For this review, take the finished solid that the model builds, in its own axes (mm). Face numbers are marked on the shaded views. A direction names the side the tool comes from. Give positions to 0.01 mm unless a question says otherwise; leave off trailing zeros. Write each loop counter-clockwise with the first axis right and the second up, starting at its lowest first coordinate (ties: lowest second). Pieces come first, ordered by that corner, then holes.
Q1. We need section B-B (z = 0). Write out the cut boundary in (x, y), then the cut area to 3 significant figures.
Q2. We need section A-A (x = 0). Write out the cut boundary in (y, z).
Q3. We need section C-C (y = -8.75). Write out the cut boundary in (x, z).
Q4. Machinability: for the marked faces 4, 5 and 6, which of the approach directions +Z, -Z, +X, -X, +Y, -Y give a long, thin tool a straight path to every point of the face, cutting with its end or side? Answer none if there is none.
Q5. For line 1 (Y direction, x = -1.3, z = -0.05); line 2 (Z direction, x = -0.1, y = -8); line 3 (Y direction, x = 1.35, z = 0.9), list the stretches that pass through material, from the lowest coordinate up.
Q6. Insertion check: P1, Ø2, axis at y = -8, z = -2, coming from the -X side; P2, Ø1.1, axis at y = 1.5, z = -1, coming from the -X side; P3, Ø1.1, axis at x = 1, y = 1.5, coming from the -Z side. Each pin has a flat end and moves straight along its axis. Give the tip position at first contact, or say it passes through.
Q7. Mouldability with a two-part tool opening along Z and no side actions: class the marked faces 1, 2 and 3 as released by +Z, released by -Z, zero draft, split by the parting line, or undercut.
Autodesk Inventor part; units mm, degrees
ref_plane "YZ Plane" through (0, 0, 0) normal (1, 0, 0) x (0, 1, 0)
ref_plane "XZ Plane" through (0, 0, 0) normal (0, 1, 0) x (-1, 0, 0)
ref_plane "XY Plane" through (0, 0, 0) normal (0, 0, 1) x (1, 0, 0)
sketch "Skizze1" plane through (0, 0, 0) normal (0, 1, 0) x (-1, 0, 0)
  circle A0 centre (0, 0) radius 2.5
  dimension "d0" = 5
extrude "Extrusion1" add sketch "Skizze1" along normal blind 2
sketch "Skizze2" plane through (0, 2, 0) normal (0, 1, 0) x (1, 0, 0)
  line L0 (-0.5, -3.2562) -> (0.5, -3.2562)
  line L1 (0.5, -3.2562) -> (0.5, 3.274)
  line L2 (0.5, 3.274) -> (-0.5, 3.274)
  line L3 (-0.5, 3.274) -> (-0.5, -3.2562)
  line L4 (1.5, -0.5) -> (-1.5, -0.5)
  line L5 (-1.5, -0.5) -> (-1.5, 0.5)
  line L6 (-1.5, 0.5) -> (1.5, 0.5)
  line L7 (1.5, 0.5) -> (1.5, -0.5)
  point P0 (0, 0)
  dimension "d3" = 1
  dimension "d4" = 1
  dimension "d5" = 0.5
  dimension "d6" = 0.5
  dimension "d7" = 3
  dimension "d8" = 1.5
fillet "Rundung1" radius 0.7 2 edges at (2.5, 2, 0) (2.5, 0, 0)
extrude "Extrusion2" cut sketch "Skizze2" against normal blind 1
sketch "Skizze3" plane through (0, 0, 0) normal (0, -1, 0) x (1, 0, 0)
  circle A0 centre (0, 0) radius 1.5
  dimension "d12" = 3
extrude "Extrusion3" add sketch "Skizze3" along normal blind 10.5
properties part number "Schraube"
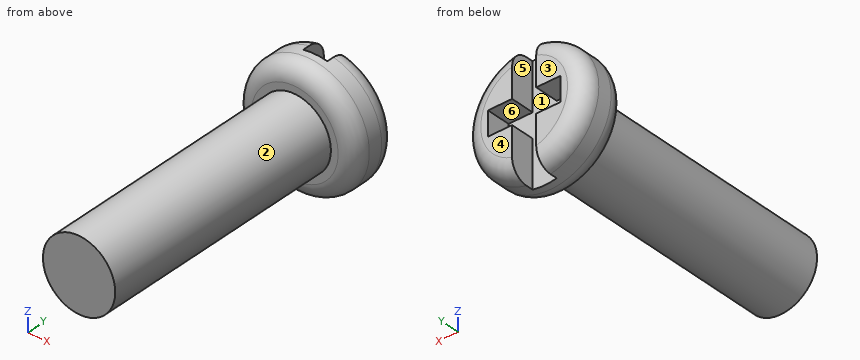
Computed:
1. outline: (-2.5, 0.7) arc R0.7 ccw to (-1.8, 0) - (-1.5, 0) - (-1.5, -10.5) - (1.5, -10.5) - (1.5, 0) - (1.8, 0) arc R0.7 ccw to (2.5, 0.7) - (2.5, 1.3) arc R0.7 ccw to (1.8, 2) - (1.5, 2) - (1.5, 1) - (-1.5, 1) - (-1.5, 2) - (-1.8, 2) arc R0.7 ccw to (-2.5, 1.3) - close
1. area: 38.1 mm2
2. outline: (-10.5, -1.5) - (0, -1.5) - (0, -1.8) arc R0.7 ccw to (0.7, -2.5) - (1, -2.5) - (1, 2.5) - (0.7, 2.5) arc R0.7 ccw to (0, 1.8) - (0, 1.5) - (-10.5, 1.5) - close
3. outline: circle Ø3 at (0, 0)
4. face 4: +Z, -Z, +X, -X, +Y
4. face 5: +Z, -Z, +Y
4. face 6: +Y
5. line 1: y = -10.5 to 1
5. line 2: z = -1.5 to 1.5
5. line 3: y = 0 to 2
6. P1: stops at x = -1.12
6. P2: stops at x = -2.45
6. P3: stops at z = -2.45
7. face 1: undercut
7. face 2: split by the parting line
7. face 3: zero draft
